```python
from build123d import *

# Parameters (mm, degrees)
F1_DEPTH = 12.7
F2_DEPTH = 12.7
F3_R     = 19.05
F4_DEPTH = 25.401
F5_R     = 7.9375
F6_DEPTH = 25.401


with BuildPart() as f1:
    # F0 (on Front) → F1 (new body, symmetric)
    with BuildSketch(Plane.XZ):
        with BuildLine():
            ThreePointArc((23.178504, -21.698374), (29.529477, -11.665012), (31.75, 0))
            ThreePointArc((31.75, 0), (-11.665012, 29.529477), (-23.178504, -21.698374))
            ThreePointArc((-23.178504, -21.698374), (0, -31.75), (23.178504, -21.698374))
        make_face()
    extrude(amount=F1_DEPTH, both=True)

    # F0 (on Front) → F2 (join, symmetric)
    with BuildSketch(Plane.XZ):
        with BuildLine():
            ThreePointArc((23.178504, -21.698374), (0, -31.75), (-23.178504, -21.698374))
            Line((-23.178504, -21.698374), (-13.455255, -67.775527))
            ThreePointArc((-13.455255, -67.775527), (0, -60.325), (13.455255, -67.775527))
            Line((13.455255, -67.775527), (23.178504, -21.698374))
        make_face()
        with BuildLine():
            ThreePointArc((13.455255, -67.775527), (0, -60.325), (-13.455255, -67.775527))
            ThreePointArc((-13.455255, -67.775527), (-4.382548, -91.458077), (15.875, -76.2))
            ThreePointArc((15.875, -76.2), (15.258077, -71.817452), (13.455255, -67.775527))
        make_face()
    extrude(amount=F2_DEPTH, both=True)

    # F3 (on face) → F4 (cut, through all)
    with BuildSketch(Plane.XZ.offset(12.7)):
        Circle(F3_R)
    extrude(amount=-F4_DEPTH, mode=Mode.SUBTRACT)

    # F5 (on face) → F6 (cut, through all)
    with BuildSketch(Plane.XZ.offset(12.7)):
        with Locations((0, -76.2)):
            Circle(F5_R)
    extrude(amount=-F6_DEPTH, mode=Mode.SUBTRACT)


solid = f1.part
```
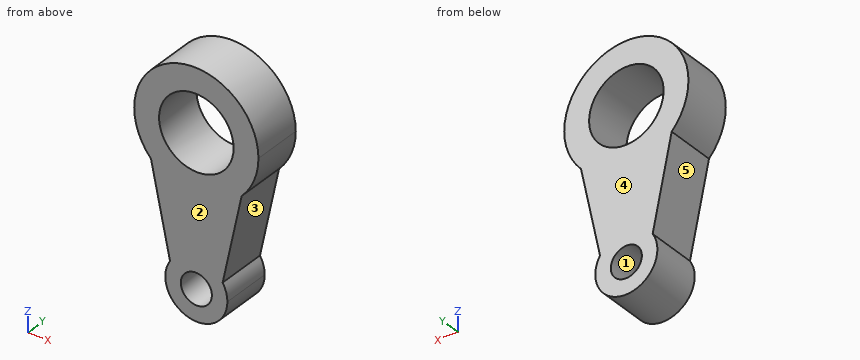
Could you check a few things on this model? Use its own coordinates, in mm. Face numbers are marked on the shaded views. A direction names the side the tool comes from. Give positions to 0.01 mm unless a question says otherwise; leave off trailing zeros. Order: outer loops, then holes, each group sorted by start corner. A loop starts at its lowest first (then second) coordinate and runs counter-clockwise, first axis right, second up.
Q1. Suppose I cut it at D-D, the plane z = -38. Write out the boundary of the cut face in (x, y).
Q2. If I drill on line 1 along Z through (x, y) = (5, 2.25); line 2 along Z through (x, y) = (13, 10.5); line 3 along X through (y, z) = (6.5, 11), over which ranges is the centre line in solid material (lowest first)?
Q3. Suppose I cut it at A-A, the plane y = 2.25. Count the separate pieces of the cut face and the enclosed holes in it, and give its area (3 significant figures).
Q4. Suppose I cut it at C-C, the plane z = -16. Write out the boundary of the cut face in (x, y).
Q5. For the marked faces 3, 4 and 5, which set-ups out of +Z, -Z, +X, -X, +Y, -Y let a thin tool reach every point of the face, with its end or its side?
Q6. I'm going to push flat-ended pins straight in: P1, Ø1.5, axis at y = -9.5, z = -67, coming from the +X side; P2, Ø1, axis at y = 6.5, z = -16, coming from the -X side; P3, Ø1.5, axis at x = -25, y = -6.5, coming from the +Z side. Where does each tip first touch, or does it pass through?
Q7. We'd pull the mould along Z, two halves only. Please class the marked faces 1 and 2: +Z half, -Z half, draft (parallel to the pull), parting line (faces both ways), or undercut.
Solution:
1. outline: (-19.74, -12.7) - (19.74, -12.7) - (19.74, 12.7) - (-19.74, 12.7) - close
2. line 1: z = -91.27 to -82.36, -70.04 to -18.38, 18.38 to 31.35
2. line 2: z = -85.31 to -13.92, 13.92 to 28.97
2. line 3: x = -29.78 to -15.55, 15.55 to 29.78
3. separate pieces: 1
3. enclosed holes: 2
3. area: 3,850 mm2
4. outline: (-27.42, -12.7) - (-10.34, -12.7) - (-10.34, 12.7) - (-27.42, 12.7) - close; (10.34, -12.7) - (27.42, -12.7) - (27.42, 12.7) - (10.34, 12.7) - close
5. face 3: +X, +Y, -Y
5. face 4: +Z, -Z, +X, -X, +Y
5. face 5: -X, +Y, -Y
6. P1: stops at x = 13.78
6. P2: stops at x = -27.71
6. P3: stops at z = 20.49
7. face 1: undercut
7. face 2: draft
